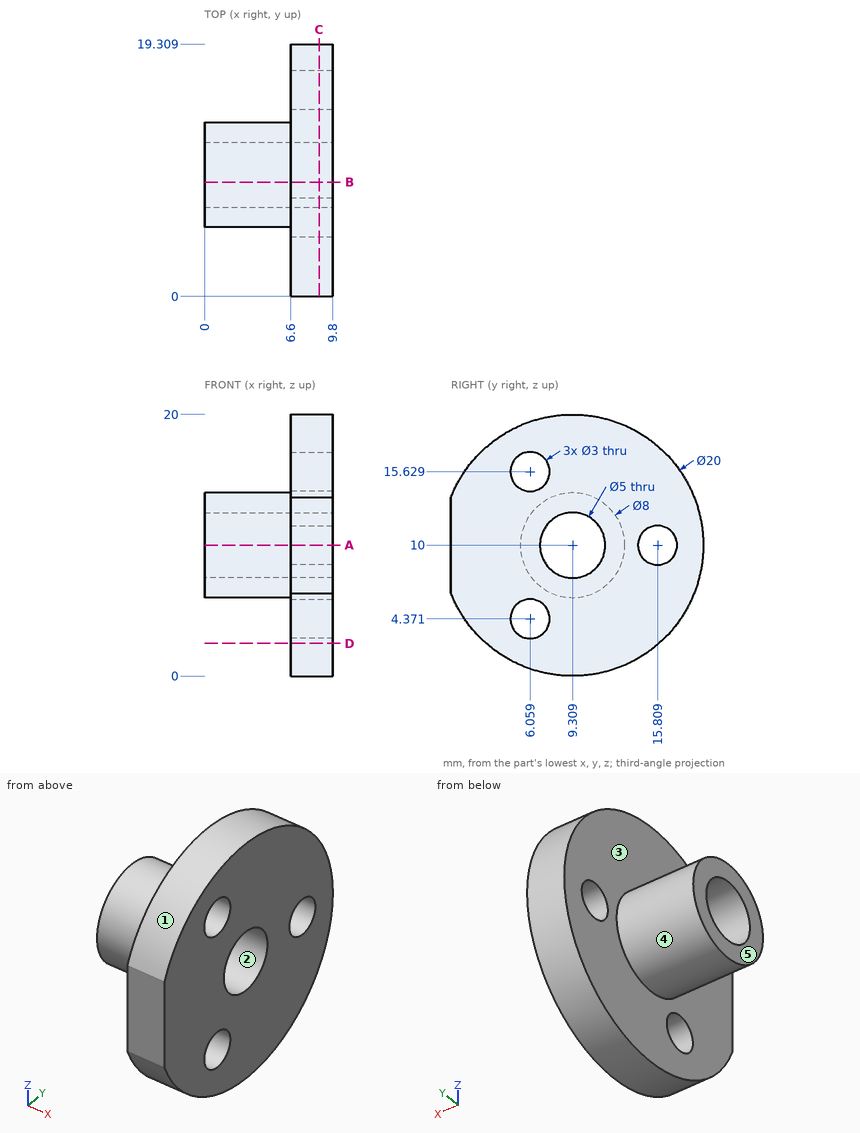
For this review, use the dimensioned drawing (mm, ordinates from the lowest corner) and the shaded views. A direction names the side the tool comes from. Coordinates: 2 decimals unless noted, no trailing zeros. Loops run counter-clockwise (first coordinate to the right, second up) from the corner with the lowest first, then second, coordinate; pieces in that order, holes last.
1. For line 1 (X direction, y = 10, z = 2.25); line 2 (Y direction, x = 7, z = 15.75) (1 decimal); line 3 (Y direction, x = 5.25, z = 10.75), list the stretches that pass through material, from the lowest coordinate up.
2. Insertion check: P1, Ø4, axis at y = 9.309, z = 10, coming from the -X side; P2, Ø4, axis at x = 5, z = 3, coming from the +Y side (1 decimal); P3, Ø4, axis at y = 2.5, z = 7, coming from the -X side; P4, Ø4, axis at x = 2, z = 9, coming from the -Y side. Each pin has a flat end and moves straight along its axis. Give the tip position at first contact, or say it passes through.
3. For the marked faces 4 and 5, list the 3-axis set-ups (+Z, -Z, +X, -X, +Y, -Y) from which the entire face can be reached by the end or side of a thin tool; tool diameter is ignored.
4. Add section A-A, the plane z = 10. Give the boundary of the cut face in (x, y).
5. Add section D-D, the plane z = 2.5. Give the boundary of the cut face in (x, y) (1 decimal), then the cut area to 3 significant figures.
6. Add section C-C, the plane x = 8.75. Give the boundary of the cut face in (y, z).
7. Add section B-B, the plane y = 8.75. Give the boundary of the cut face in (x, z).
8. Mouldability with a two-part tool opening along Y and no side actions: class the marked faces 1, 2 and 3 as +Y half, -Y half, draft (parallel to the pull), parting line (faces both ways), or undercut.
Result:
1. line 1: x = 6.6 to 9.8
1. line 2: y = 1.1 to 4.6, 7.6 to 17.5
1. line 3: y = 5.38 to 6.92, 11.69 to 13.24
2. P1: passes through
2. P2: stops at y = 17.5
2. P3: stops at x = 6.6
2. P4: stops at y = 5.31
3. face 4: -X
3. face 5: +Z, -Z, -X, +Y, -Y
4. outline: (0, 5.31) - (6.6, 5.31) - (6.6, 0) - (9.8, 0) - (9.8, 6.81) - (0, 6.81) - close; (0, 11.81) - (9.8, 11.81) - (9.8, 14.31) - (6.6, 14.31) - (6.6, 13.31) - (0, 13.31) - close; (6.6, 17.31) - (9.8, 17.31) - (9.8, 19.31) - (6.6, 19.31) - close
5. outline: (6.6, 2.7) - (9.8, 2.7) - (9.8, 15.9) - (6.6, 15.9) - close
5. area: 42.3 mm2
6. outline: (0, 6.35) arc R10 ccw (long way) to (0, 13.65) - close; hole circle Ø3 at (6.06, 4.37); hole circle Ø3 at (6.06, 15.63); hole circle Ø5 at (9.31, 10); hole circle Ø3 at (15.81, 10)
7. outline: (0, 6.04) - (6.6, 6.04) - (6.6, 0.02) - (9.8, 0.02) - (9.8, 7.56) - (0, 7.56) - close; (0, 12.44) - (9.8, 12.44) - (9.8, 19.98) - (6.6, 19.98) - (6.6, 13.96) - (0, 13.96) - close
8. face 1: parting line
8. face 2: undercut
8. face 3: draft
